from build123d import *

# Parameters (mm, degrees)
SKETCH1_W           = 210
SKETCH1_H           = 100
SKETCH1_W_2         = 190.2
SKETCH1_H_2         = 70.2
BOSS_EXTRUDE1_DEPTH = 1.5
SKETCH2_W           = 210
SKETCH2_H           = 100
SKETCH2_W_2         = 5
SKETCH2_H_2         = 5
BOSS_EXTRUDE2_DEPTH = 20


with BuildPart() as part:
    # Sketch1 → Boss-Extrude1 (new body)
    with BuildSketch(Plane.XY):
        with Locations((95.1, 35.1)):
            Rectangle(SKETCH1_W, SKETCH1_H)
        with Locations((95.1, 35.1)):
            Rectangle(SKETCH1_W_2, SKETCH1_H_2, mode=Mode.SUBTRACT)
    extrude(amount=BOSS_EXTRUDE1_DEPTH)

    # Sketch2 → Boss-Extrude2 (add)
    # profile 1 of 5: a face of its own
    with BuildSketch(Plane.XY.offset(1.5)):
        with Locations((95.1, 35.1)):
            Rectangle(SKETCH2_W, SKETCH2_H)
        Polygon((0, 65.2), (0, 70.2), (5, 70.2), (185.2, 70.2), (190.2, 70.2), (190.2, 65.2), (190.2, 5), (190.2, 0), (185.2, 0), (5, 0), (0, 0), (0, 5), align=None, mode=Mode.SUBTRACT)
    # profile 2 of 5: a face of its own
    with BuildSketch(Plane.XY.offset(1.5)):
        with Locations((2.5, 67.7)):
            Rectangle(SKETCH2_W_2, SKETCH2_H_2)
    # profile 3 of 5: a face of its own
    with BuildSketch(Plane.XY.offset(1.5)):
        with Locations((2.5, 2.5)):
            Rectangle(SKETCH2_W_2, SKETCH2_H_2)
    # profile 4 of 5: a face of its own
    with BuildSketch(Plane.XY.offset(1.5)):
        with Locations((187.7, 67.7)):
            Rectangle(SKETCH2_W_2, SKETCH2_H_2)
    # profile 5 of 5: a face of its own
    with BuildSketch(Plane.XY.offset(1.5)):
        with Locations((187.7, 2.5)):
            Rectangle(SKETCH2_W_2, SKETCH2_H_2)
    extrude(amount=BOSS_EXTRUDE2_DEPTH)


solid = part.part
The listing builds one solid part. Answer for the finished solid, in the listing's coordinates (mm). A direction names the side the tool comes from. Give positions to 0.01 mm unless a question says otherwise; leave off trailing zeros. Write each loop counter-clockwise with the first axis right and the second up, starting at its lowest first coordinate (ties: lowest second). Pieces come first, ordered by that corner, then holes.
1) Section A-A (x = 86) is taken. Write down the section's boundary in (y, z).
2) For a pull along X with two mould halves and no side action, classify faces 1 (the face through (2, 5, 11)), 2 (the face through (94, 85.1, 11)), 3 (the face through (-9.9, 34, 11)), 4 (the face through (188, 3, 1.5)) as pulls with the +X half, pulls with the -X half, needs draft (parallel to the pull), parting line crosses it, or undercut.
3) A tool of negligible diameter and unlimited length cuts with its end or side. For faces 5 (the face through (79, -2, 21.5)), 6 (the face through (2, 68, 1.5)), 7 (the face through (5, 68, 11)), from which of +Z, -Z, +X, -X, +Y, -Y can it reach the whole face along a straight path? Write none if from no direction.
4) Section C-C (z = 7.5) is taken. Write down the section's boundary in (x, y), and give its area (3 significant figures).
5) Given P1, Ø1.5, axis at x = 1.5, y = 1.5, coming from the -Z side, flat-ended and moving along its own axis, determine where the tip first touches the part or whether it passes through.
6) Section B-B (y = 41) is taken. Write down the section's boundary in (x, z).
7) Find the intervals of material crossed by L1, parallel to Y at x = 101, z = 10.25; L2, parallel to X at y = 40.5, z = 12.5, in increasing order.
Response:
1. outline: (-14.9, 0) - (0, 0) - (0, 21.5) - (-14.9, 21.5) - close; (70.2, 0) - (85.1, 0) - (85.1, 21.5) - (70.2, 21.5) - close
2. face 1: undercut
2. face 2: needs draft
2. face 3: pulls with the -X half
2. face 4: undercut
3. face 5: +Z, +X, -X, +Y, -Y
3. face 6: -Z
3. face 7: +Z, -Z
4. outline: (-9.9, -14.9) - (200.1, -14.9) - (200.1, 85.1) - (-9.9, 85.1) - close; hole (0, 5) - (5, 5) - (5, 0) - (185.2, 0) - (185.2, 5) - (190.2, 5) - (190.2, 65.2) - (185.2, 65.2) - (185.2, 70.2) - (5, 70.2) - (5, 65.2) - (0, 65.2) - close
4. area: 7,750 mm2
5. P1: stops at z = 1.5
6. outline: (-9.9, 0) - (0, 0) - (0, 21.5) - (-9.9, 21.5) - close; (190.2, 0) - (200.1, 0) - (200.1, 21.5) - (190.2, 21.5) - close
7. L1: y = -14.9 to 0, 70.2 to 85.1
7. L2: x = -9.9 to 0, 190.2 to 200.1
